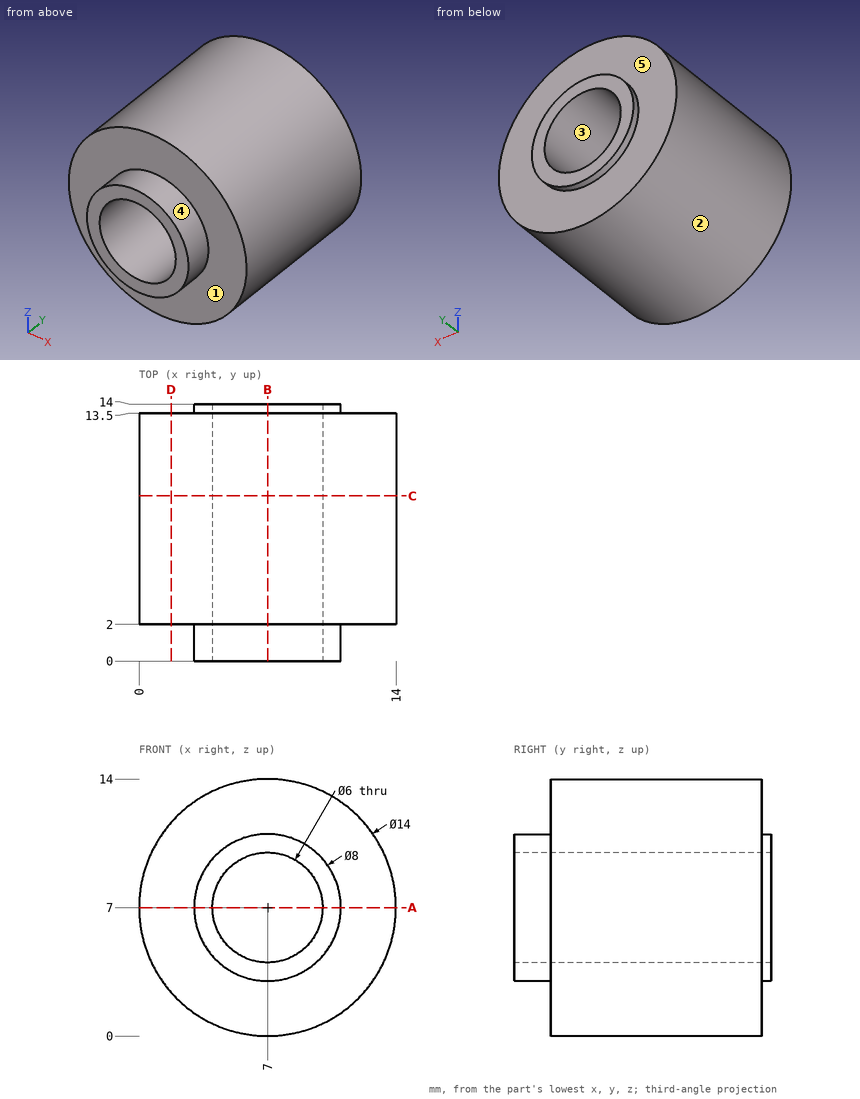
Source: three-view drawing plus pictorial views. Frame: mm from the lowest corner of the part. A direction names the side the tool comes from. Round coordinates to 2 decimals unless told otherwise and drop trailing zeros. Loops run counter-clockwise (first coordinate to the right, second up) from the corner with the lowest first, then second, coordinate; pieces in that order, holes last. Notation, with made-up numbers: (33.25, 89) - (45.25, 89) arc R8 ccw to (45.25, 94) - close; hole circle Ø7 at (22, 53.25). An arc over 180 degrees is marked (long way). Write item = value, one per line. Start each with the question number.
Item 1: Section query B-B on x = 7. Output: boundary loops of the cut face in (y, z), plus the area to 3 significant figures.
Item 2: Section query A-A on z = 7. Output: boundary loops of the cut face in (x, y).
Item 3: Section query C-C on y = 9. Output: boundary loops of the cut face in (x, z), plus the area to 3 significant figures.
Item 4: Mould query, pull axis Z, two halves, no side actions, for the marked faces 1, 2 and 3. Classes: released by +Z, released by -Z, zero draft, split by the parting line, or undercut.
Item 5: First-contact query: pin 1 Ø1.5 at (x, y) = (5.5, 10) entering from -Z; pin 2 Ø2 at (x, y) = (4.5, 5) entering from +Z. Flat tips, straight axial feed; report the tip coordinate or a pass-through.
Item 6: Section query D-D on x = 1.75. Output: boundary loops of the cut face in (y, z).
Item 7: Material intervals for line 1 (X direction, y = 11, z = 7); line 2 (X direction, y = 1.75, z = 7); line 3 (Y direction, x = 4.75, z = 3.25), sorted ascending.
Item 8: Reachability of the marked faces 4 and 5 from +Z, -Z, +X, -X, +Y, -Y: full face, straight path, thin tool, end or side. Return the list, or none.
Results list:
q1.outline = (0, 3) - (2, 3) - (2, 0) - (13.5, 0) - (13.5, 3) - (14, 3) - (14, 4) - (0, 4) - close; (0, 10) - (14, 10) - (14, 11) - (13.5, 11) - (13.5, 14) - (2, 14) - (2, 11) - (0, 11) - close
q1.area = 97.0 mm²
q2.outline = (0, 2) - (3, 2) - (3, 0) - (4, 0) - (4, 14) - (3, 14) - (3, 13.5) - (0, 13.5) - close; (10, 0) - (11, 0) - (11, 2) - (14, 2) - (14, 13.5) - (11, 13.5) - (11, 14) - (10, 14) - close
q3.outline = circle Ø14 at (7, 7); hole circle Ø6 at (7, 7)
q3.area = 126 mm²
q4.face_1 = zero draft
q4.face_2 = split by the parting line
q4.face_3 = undercut
q5.pin_1 = 0.04
q5.pin_2 = 13.84
q6.outline = (2, 2.37) - (13.5, 2.37) - (13.5, 11.63) - (2, 11.63) - close
q7.line_1 = 0 to 4, 10 to 14
q7.line_2 = 3 to 4, 10 to 11
q7.line_3 = 2 to 13.5
q8.face_4 = -Y
q8.face_5 = +Y
